Geometry check sheet. Reference: the model listing, model coordinates, mm. Face numbers are marked on the shaded views. A direction names the side the tool comes from. Round coordinates to 2 decimals unless told otherwise and drop trailing zeros. Write each loop counter-clockwise with the first axis right and the second up, starting at its lowest first coordinate (ties: lowest second). Pieces come first, ordered by that corner, then holes. Notation, with made-up numbers: M 18,21.25 L 23,21.25 A23 cw 23,59.25 Z; hole C -38.5,-11.75 d8. An arc over 180 degrees is marked long. One line per item, written item: value. Start each with the question number.
1. Section check A-A (y = 10.5). Record the boundary of the cut face in (x, z), and give its area (3 significant figures).
2. Scan lines: probe 1 along Z at (x, y) = (-5.5, 29.5); probe 2 along Z at (x, y) = (23, 6); probe 3 along X at (y, z) = (13, 20.5). Record each from-to range of solid material in increasing order. Write a range as [from, to].
3. Section check B-B (z = 25). Record the boundary of the cut face in (x, y), and give its area (3 significant figures).
4. Depth check by flat-ended pin: P1, Ø4, axis at y = -27.5, z = 26.5, coming from the -X side; P2, Ø1.5, axis at x = 1.5, y = 9, coming from the +Z side; P3, Ø6, axis at x = 36.5, y = 4.5, coming from the +Z side. Enter the tip coordinate at first touch or a pass-through.
5. Access from +Z, -Z, +X, -X, +Y, -Y to the whole of each face (thin tool, end or side, straight path). Record for the marked faces 1 and 2.
6. Section check C-C (x = 17). Record the boundary of the cut face in (y, z), and give its area (3 significant figures).
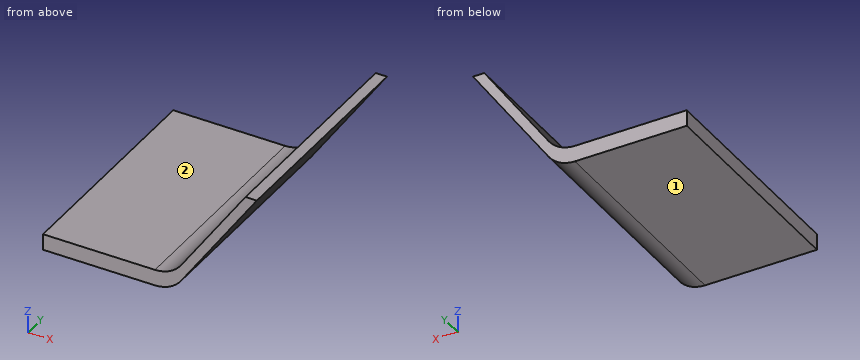
from build123d import *

# Parameters (mm, degrees)
F0_W     = 40
F0_H     = 70
F1_DEPTH = 5
F3_DEPTH = 35
F4_R     = 10


with BuildPart() as f1:
    # F0 (on Top) → F1 (new body)
    with BuildSketch(Plane.XY):
        Rectangle(F0_W, F0_H)
    extrude(amount=F1_DEPTH)

    # F2 (on Front) → F3 (join, symmetric)
    with BuildSketch(Plane.XZ):
        Polygon((42.943057, 37.766082), (20, 5), (20, 0), (46.444095, 37.766082), align=None)
    extrude(amount=F3_DEPTH, both=True)

    # F4
    f4_edges = [f1.edges().sort_by_distance(p)[0] for p in [
        (20, 0, 5),
        (20, 0, 0),
    ]]
    fillet(f4_edges, radius=F4_R)


solid = f1.part
Result sheet:
1. outline: M -20,0 L 14.79,0 A10 ccw 22.99,4.26 L 46.44,37.77 L 42.94,37.77 L 22.99,9.26 A10 cw 14.79,5 L -20,5 Z
1. area: 323 mm2
2. probe 1: z = [0, 5]
2. probe 2: z = [4.28, 9.28]
2. probe 3: x = [30.85, 34.35]
3. outline: M 34,-35 L 37.51,-35 L 37.51,35 L 34,35 Z
3. area: 245 mm2
4. P1: stops at x = 33.65
4. P2: stops at z = 5
4. P3: stops at z = 32.85
5. face 1: -Z, +X, -X, +Y, -Y
5. face 2: +Z, -X, +Y, -Y
6. outline: M -35,0.25 L 35,0.25 L 35,5.25 L -35,5.25 Z
6. area: 350 mm2
